from build123d import *

# Parameters (mm, degrees)
SKETCH_1_R      = 1.5
EXTRUDE_1_DEPTH = 10
EXTRUDE_2_DEPTH = 2
SKETCH_3_R      = 1.5
EXTRUDE_3_DEPTH = 5


with BuildPart() as part:
    # 草图1 → 凸台-拉伸1 (new body)
    with BuildSketch(Plane.XY):
        Polygon((0, 2.424871131), (-2.1, 1.212435565), (-2.1, -1.212435565), (0, -2.424871131), (2.1, -1.212435565), (2.1, 1.212435565), align=None)
        Circle(SKETCH_1_R, mode=Mode.SUBTRACT)
    extrude(amount=EXTRUDE_1_DEPTH)

    # 草图2 → 凸台-拉伸2 (add)
    with BuildSketch(Plane.XY.offset(10)):
        Polygon((2.1, 1.212435565), (0, 2.424871131), (-2.1, 1.212435565), (-2.1, -1.212435565), (0, -2.424871131), (2.1, -1.212435565), align=None)
    extrude(amount=EXTRUDE_2_DEPTH)

    # 草图3 → 凸台-拉伸3 (add)
    with BuildSketch(Plane.XY.offset(12)):
        Circle(SKETCH_3_R)
    extrude(amount=EXTRUDE_3_DEPTH)


solid = part.part
Geometry: final body of the model. Coordinates: model frame, mm. A direction names the side the tool comes from. Coordinates: 2 decimals unless noted, no trailing zeros. Order: outer loops, then holes, each group sorted by start corner. A loop starts at its lowest first (then second) coordinate and runs counter-clockwise, first axis right, second up.
1) Section A-A (y = 0). Return loops of the section in (x, z).
Result sheet:
outline: (-2.1, 0) - (-1.5, 0) - (-1.5, 10) - (1.5, 10) - (1.5, 0) - (2.1, 0) - (2.1, 12) - (1.5, 12) - (1.5, 17) - (-1.5, 17) - (-1.5, 12) - (-2.1, 12) - close
2) First-contact query: P1, Ø1, axis at x = 1.5, z = 8.5, coming from the +Y side; P2, Ø2.5, axis at x = 0, y = 0, coming from the -Z side; P3, Ø1.5, axis at x = 1.5, z = 11.5, coming from the -Y side. Flat tips, straight axial feed; report the tip coordinate or a pass-through.
Result sheet:
P1: stops at y = 1.85
P2: stops at z = 10
P3: stops at y = -1.99
3) Draft query along Y for faces 1 (the flat face through (-1.065, -1.81, 5.916)), 2 (the flat face through (0, 0, 10)), 3 (the flat face through (0, 0, 17)). Return one class per face: released by +Y, released by -Y, zero draft, split by the parting line, or undercut.
Result sheet:
face 1: released by -Y
face 2: undercut
face 3: zero draft
4) Section B-B (z = 11.5). Return loops of the section in (x, y), then the cut area to 3 significant figures.
Result sheet:
outline: (-2.1, -1.21) - (0, -2.42) - (2.1, -1.21) - (2.1, 1.21) - (0, 2.42) - (-2.1, 1.21) - close
area: 15.3 mm2
5) Section C-C (x = -0.7). Return loops of the section in (y, z), then the cut area to 3 significant figures.
Result sheet:
outline: (-2.02, 0) - (-1.33, 0) - (-1.33, 10) - (1.33, 10) - (1.33, 0) - (2.02, 0) - (2.02, 12) - (1.33, 12) - (1.33, 17) - (-1.33, 17) - (-1.33, 12) - (-2.02, 12) - close
area: 35.2 mm2
6) Set-up query: faces 4 (the cylindrical face through (-1.5, 0.07, 14.46)), 5 (the flat face through (2.1, 0, 6)), 6 (the cylindrical face through (-1.5, 0.07, 4.93)). Return all of +Z, -Z, +X, -X, +Y, -Y with unobstructed straight access to the full face (end or side cutting, diameter ignored); none if empty.
Result sheet:
face 4: +Z
face 5: +Z, -Z, +X, +Y, -Y
face 6: -Z
7) Section D-D (z = 14). Return loops of the section in (x, y), then the cut area to 3 significant figures.
Result sheet:
outline: circle Ø3 at (0, 0)
area: 7.07 mm2
8) Ray query, probe 1 along Z at (x, y) = (0.15, -2); probe 2 along Y at (x, z) = (0.5, 1); probe 3 along Y at (x, z) = (0.7, 3.5). Return the intervals inside material, ascending.
Result sheet:
probe 1: z = 0 to 12
probe 2: y = -2.14 to -1.41, 1.41 to 2.14
probe 3: y = -2.02 to -1.33, 1.33 to 2.02
